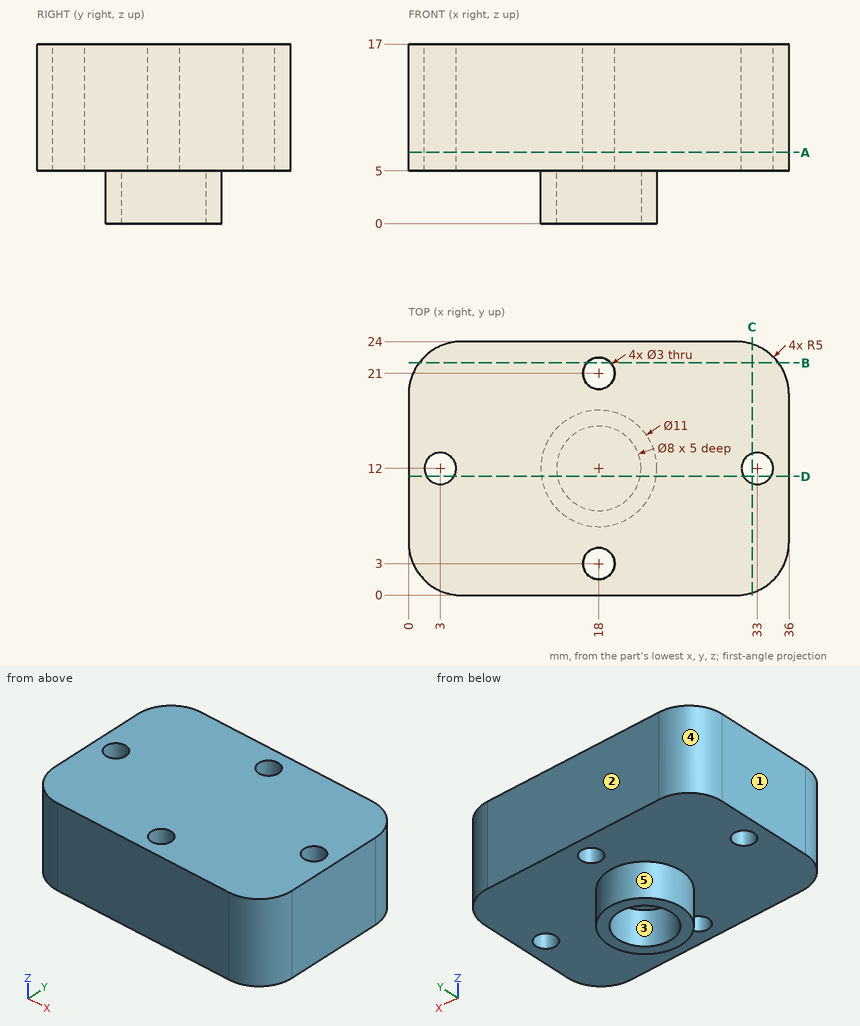
Here's the drawing with two shaded views (mm, measured from the low corner). I have some questions. A direction names the side the tool comes from. Give positions to 0.01 mm unless a question says otherwise; leave off trailing zeros. Order: outer loops, then holes, each group sorted by start corner. A loop starts at its lowest first (then second) coordinate and runs counter-clockwise, first axis right, second up.
Q1. Suppose I cut it at B-B, the plane y = 22. Write out the boundary of the cut face in (x, z).
Q2. Suppose I cut it at D-D, the plane y = 11.25. Write out the boundary of the cut face in (x, z), and give its area (3 significant figures).
Q3. If I drill on line 1 along X through (y, z) = (12, 9.5); line 2 along Y through (x, z) = (18, 10); line 3 along Z through (x, y) = (23.5, 10.5), over which ranges is the centre line in solid material (lowest first)?
Q4. We'd pull the mould along X, two halves only. Please class the marked faces 1, 2 and 3: +X half, -X half, draft (parallel to the pull), parting line (faces both ways), or undercut.
Q5. For the marked faces 4 and 5, which set-ups out of +Z, -Z, +X, -X, +Y, -Y let a thin tool reach every point of the face, with its end or its side?
Q6. Suppose I cut it at C-C, the plane x = 32.5. Write out the boundary of the cut face in (y, z), and give its area (3 significant figures).
Q7. Suppose I cut it at A-A, the plane z = 6.75. Write out the boundary of the cut face in (x, y).
Q8. I'm going to push flat-ended pins straight in: P1, Ø2.5, axis at x = 18, y = 3, coming from the +Z side; P2, Ø1.5, axis at y = 13, z = 4, coming from the +X side; P3, Ø6.5, axis at x = 18, y = 12, coming from the -Z side; P4, Ø1, axis at y = 3.5, z = 9, coming from the +X side. Where does each tip first touch, or does it pass through?
Solution:
1. outline: (1, 5) - (16.88, 5) - (16.88, 17) - (1, 17) - close; (19.12, 5) - (35, 5) - (35, 17) - (19.12, 17) - close
2. outline: (0, 5) - (1.7, 5) - (1.7, 17) - (0, 17) - close; (4.3, 5) - (12.55, 5) - (12.55, 0) - (14.07, 0) - (14.07, 5) - (21.93, 5) - (21.93, 0) - (23.45, 0) - (23.45, 5) - (31.7, 5) - (31.7, 17) - (4.3, 17) - close; (34.3, 5) - (36, 5) - (36, 17) - (34.3, 17) - close
2. area: 385 mm2
3. line 1: x = 0 to 1.5, 4.5 to 31.5, 34.5 to 36
3. line 2: y = 0 to 1.5, 4.5 to 19.5, 22.5 to 24
3. line 3: z = 5 to 17
4. face 1: -X half
4. face 2: draft
4. face 3: undercut
5. face 4: +Z, -Z, -X, +Y
5. face 5: -Z
6. outline: (0.23, 5) - (10.59, 5) - (10.59, 17) - (0.23, 17) - close; (13.41, 5) - (23.77, 5) - (23.77, 17) - (13.41, 17) - close
6. area: 249 mm2
7. outline: (0, 5) arc R5 ccw to (5, 0) - (31, 0) arc R5 ccw to (36, 5) - (36, 19) arc R5 ccw to (31, 24) - (5, 24) arc R5 ccw to (0, 19) - close; hole circle Ø3 at (3, 12); hole circle Ø3 at (18, 3); hole circle Ø3 at (18, 21); hole circle Ø3 at (33, 12)
8. P1: passes through
8. P2: stops at x = 23.49
8. P3: stops at z = 5
8. P4: stops at x = 35.9
